from build123d import *

# Parameters (mm, degrees)
BOSS_EXTRUDE1_DEPTH      = 25.4
BOSS_EXTRUDE1_DEPTH_BACK = 25.4
SKETCH2_W                = 50.8
SKETCH2_H                = 25.4
CUT_EXTRUDE1_DEPTH       = 51.8
SKETCH3_R                = 6.35
CUT_EXTRUDE2_DEPTH       = 1
CUT_EXTRUDE2_DEPTH_BACK  = 26.4


with BuildPart() as part:
    # Sketch1 → Boss-Extrude1 (new body, two sides)
    with BuildSketch(Plane.XY) as boss_extrude1_sk:
        Polygon((0, 0), (0, 50.8), (6.35, 50.8), (6.35, 6.35), (50.8, 6.35), (50.8, 0), align=None)
    extrude(amount=BOSS_EXTRUDE1_DEPTH)
    extrude(boss_extrude1_sk.sketch, amount=-BOSS_EXTRUDE1_DEPTH_BACK)

    # Sketch2 → Cut-Extrude1 (cut, through all)
    with BuildSketch(Plane.ZY):
        with Locations((0, 38.1)):
            Rectangle(SKETCH2_W, SKETCH2_H)
    extrude(amount=-CUT_EXTRUDE1_DEPTH, mode=Mode.SUBTRACT)

    # Sketch3 → Cut-Extrude2 (cut, two sides)
    with BuildSketch(Plane.XZ) as cut_extrude2_sk:
        with Locations((25.4, 0)):
            Circle(SKETCH3_R)
    extrude(amount=CUT_EXTRUDE2_DEPTH, mode=Mode.SUBTRACT)
    extrude(cut_extrude2_sk.sketch, amount=-CUT_EXTRUDE2_DEPTH_BACK, mode=Mode.SUBTRACT)


solid = part.part
Read the model definition and answer for the solid it produces. Units are mm, in the model's axes. A direction names the side the tool comes from. Coordinates: 2 decimals unless noted, no trailing zeros. Order: outer loops, then holes, each group sorted by start corner. A loop starts at its lowest first (then second) coordinate and runs counter-clockwise, first axis right, second up. Notation, with made-up numbers: M 86,1.25 L 124,1.25 A24 ccw 124,19.25 Z; hole C 57,-15 d11. An arc over 180 degrees is marked long. Put each result on its own line as item: value. Start each with the question number.
Item 1: Section A-A, the plane z = 0 is taken. Determine the outline of the cut face in (x, y), plus the area to 3 significant figures.
Item 2: Given pin 1 Ø10 at (y, z) = (15.5, 10.5) entering from +X, flat-ended and moving along its own axis, determine where the tip first touches the part or whether it passes through.
Item 3: Consider probe 1 along Z at (x, y) = (25.4, 3); probe 2 along Y at (x, z) = (26, 15). Determine where each line is inside the solid, lowest interval first. Write a range as [from, to].
Item 4: For faces 4 (the face through (20, 0, 6)), 5 (the face through (6.35, 16, 0)), determine the directions among +Z, -Z, +X, -X, +Y, -Y from which every point of the face is accessible in a straight line to the end or side of a thin tool.
Item 5: Section B-B, the plane x = 25.4 is taken. Determine the outline of the cut face in (y, z).
Item 6: Section C-C, the plane z = -15.5 is taken. Determine the outline of the cut face in (x, y).
Item 7: The mould has two halves that part along Z. Classify faces 1 (the face through (0, 13, 0)), 2 (the face through (19.056, 3.131, 0.279)), 3 (the face through (20, 5, -25.4)): +Z half, -Z half, draft (parallel to the pull), parting line (faces both ways), or undercut.
Item 8: Section D-D, the plane x = 15 is taken. Determine the outline of the cut face in (y, z), plus the area to 3 significant figures.
Computed:
1. outline: M 0,0 L 19.05,0 L 19.05,6.35 L 6.35,6.35 L 6.35,25.4 L 0,25.4 Z; M 31.75,0 L 50.8,0 L 50.8,6.35 L 31.75,6.35 Z
1. area: 363 mm2
2. pin 1: stops at x = 6.35
3. probe 1: z = [-25.4, -6.35], [6.35, 25.4]
3. probe 2: y = [0, 6.35]
4. face 4: +Z, -Z, +X, -X, -Y
4. face 5: +Z, -Z, +X, +Y
5. outline: M 0,-25.4 L 6.35,-25.4 L 6.35,-6.35 L 0,-6.35 Z; M 0,6.35 L 6.35,6.35 L 6.35,25.4 L 0,25.4 Z
6. outline: M 0,0 L 50.8,0 L 50.8,6.35 L 6.35,6.35 L 6.35,25.4 L 0,25.4 Z
7. face 1: draft
7. face 2: undercut
7. face 3: -Z half
8. outline: M 0,-25.4 L 6.35,-25.4 L 6.35,25.4 L 0,25.4 Z
8. area: 323 mm2
